Could you check a few things on this model? Use its own coordinates, in mm. Coordinates: 2 decimals unless noted, no trailing zeros. Loops run counter-clockwise (first coordinate to the right, second up) from the corner with the lowest first, then second, coordinate; pieces in that order, holes last. Notation, with made-up numbers: (84.5, 20) -> (98.5, 20) arc R34 cw to (98.5, 51) -> close; hole circle Ø1 at (-13, 82). An arc over 180 degrees is marked (long way). One line per question, with ' | ' between items. Start each with the question number.
(1) If I drill on line 1 along Y through (x, z) = (0, 1.4); line 2 along X through (y, z) = (80, 1.7); line 3 along Y through (x, z) = (10, 0.8), over which ranges is the centre line in solid material (lowest first)?
(2) Suppose I cut it at C-C (y = 58). Please give me the cut outline in (x, z), plus the area to 3 significant figures.
(3) Suppose I cut it at D-D (x = -26.5). Please give me the cut outline in (y, z), plus the area to 3 significant figures.
(4) Suppose I cut it at B-B (z = 0.5). Give the number of separate pieces and of enclosed holes in the cut face, plus the area to 3 significant figures.
(5) Suppose I cut it at A-A (x = 49). Please give me the cut outline in (y, z), plus the area to 3 significant figures.
(6) I'm going to push flat-ended pins straight in: pin 1 Ø1 at (y, z) = (24, 0.5) entering from +X; pin 2 Ø3 at (x, y) = (-8.79, 130.15) entering from -Z; pin 3 Ø1 at (y, z) = (41, 1) entering from +X; pin 4 Ø1 at (x, z) = (10, 1.5) entering from +Y. Where does each tip first touch, or does it pass through?
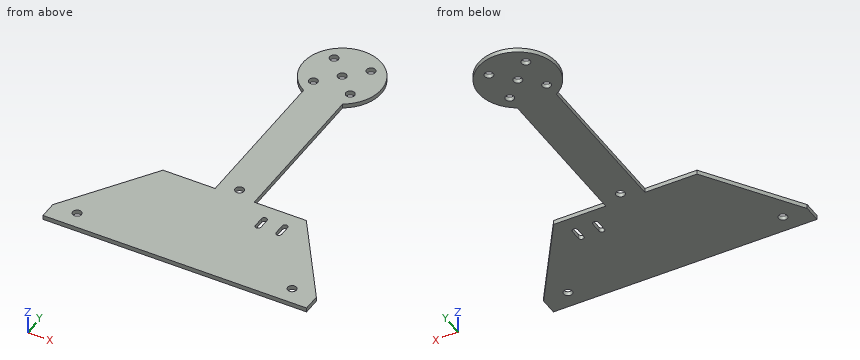
```python
from build123d import *

# Parameters (mm, degrees)
SKETCH_1_R      = 2
EXTRUDE_1_DEPTH = 2


with BuildPart() as part:
    # 草图1 → 凸台-拉伸1 (new body)
    with BuildSketch(Plane.XY):
        with BuildLine():
            Line((-9.291428571, 106.057257018), (-9.291428571, 33.645714286))
            Line((-9.291428571, 33.645714286), (-33.291428571, 33.645714286))
            Line((-33.291428571, 33.645714286), (-60.986481548, -7.354285714))
            Line((-60.986481548, -7.354285714), (-60.986481548, -15.354285714))
            Line((-60.986481548, -15.354285714), (60.403624405, -15.354285714))
            Line((60.403624405, -15.354285714), (60.403624405, -7.354285714))
            Line((60.403624405, -7.354285714), (32.708571429, 33.645714286))
            Line((32.708571429, 33.645714286), (8.708571429, 33.645714286))
            Line((8.708571429, 33.645714286), (8.708571429, 106.057257018))
            ThreePointArc((8.708571429, 106.057257018), (-0.291428571, 139.645714286), (-9.291428571, 106.057257018))
        make_face()
        with Locations((-49.791428571, -7.354285714)):
            Circle(SKETCH_1_R, mode=Mode.SUBTRACT)
        with Locations((-0.291428571, 37.645714286)):
            Circle(SKETCH_1_R, mode=Mode.SUBTRACT)
        with Locations((49.208571429, -7.354285714)):
            Circle(SKETCH_1_R, mode=Mode.SUBTRACT)
        with BuildLine():
            ThreePointArc((16.453130984, 25.945714286), (17.703130984, 27.195714286), (18.953130984, 25.945714286))
            Line((18.953130984, 25.945714286), (18.953130984, 20.945714286))
            ThreePointArc((18.953130984, 20.945714286), (17.703130984, 19.695714286), (16.453130984, 20.945714286))
            Line((16.453130984, 20.945714286), (16.453130984, 25.945714286))
        make_face(mode=Mode.SUBTRACT)
        with BuildLine():
            ThreePointArc((25.953130984, 25.945714286), (27.203130984, 27.195714286), (28.453130984, 25.945714286))
            Line((28.453130984, 25.945714286), (28.453130984, 20.945714286))
            ThreePointArc((28.453130984, 20.945714286), (27.203130984, 19.695714286), (25.953130984, 20.945714286))
            Line((25.953130984, 20.945714286), (25.953130984, 25.945714286))
        make_face(mode=Mode.SUBTRACT)
        with Locations((8.208571429, 130.145714286)):
            Circle(SKETCH_1_R, mode=Mode.SUBTRACT)
        with Locations((-8.791428571, 113.145714286)):
            Circle(SKETCH_1_R, mode=Mode.SUBTRACT)
        with Locations((-0.291428571, 121.645714286)):
            Circle(SKETCH_1_R, mode=Mode.SUBTRACT)
        with Locations((-8.791428571, 130.145714286)):
            Circle(SKETCH_1_R, mode=Mode.SUBTRACT)
        with Locations((8.208571429, 113.145714286)):
            Circle(SKETCH_1_R, mode=Mode.SUBTRACT)
    extrude(amount=EXTRUDE_1_DEPTH)


solid = part.part
```
Checks:
1) line 1: y = -15.35 to 35.67, 39.62 to 119.67, 123.62 to 139.64 | line 2: x = -9.29 to 8.71 | line 3: y = -15.35 to 33.65, 106.88 to 112.26, 114.03 to 129.26, 131.03 to 136.41
2) outline: (-9.29, 0) -> (8.71, 0) -> (8.71, 2) -> (-9.29, 2) -> close | area: 36.0 mm^2
3) outline: (-15.35, 0) -> (33.65, 0) -> (33.65, 2) -> (-15.35, 2) -> close | area: 98.0 mm^2
4) separate pieces: 1 | enclosed holes: 10 | area: 6,970 mm^2
5) outline: (-15.35, 0) -> (-9.34, 0) -> (-9.34, 2) -> (-15.35, 2) -> close; (-5.37, 0) -> (9.53, 0) -> (9.53, 2) -> (-5.37, 2) -> close | area: 41.8 mm^2
6) pin 1: stops at x = 39.56 | pin 2: passes through | pin 3: stops at x = 8.71 | pin 4: stops at y = 136.75
